Read the model definition and answer for the solid it produces. Units are mm, in the model's axes. A direction names the side the tool comes from. Give positions to 0.01 mm unless a question says otherwise; leave off trailing zeros. Order: outer loops, then holes, each group sorted by start corner. A loop starts at its lowest first (then second) coordinate and runs counter-clockwise, first axis right, second up. Notation, with made-up numbers: (44.25, -3.75) - (103.25, -3.75) arc R20 cw to (103.25, 25.25) - close; hole circle Ø4 at (71.25, -36). An arc over 180 degrees is marked (long way). Use a Markdown table: item, result. Add a question column.
1. Consider L1, parallel to Z at x = 25, y = 6.56; L2, parallel to Z at x = 13.5, y = 30.5; L3, parallel to Y at x = 27.5, z = -15 (3 decimals). Determine where each line is inside the solid, lowest interval first.
2. Which of the six approach directions +Z, -Z, +X, -X, +Y, -Y give full straight-line access (tool end or side, diameter ignored) to faces 1 (the flat face through (20, 8, -20)), 2 (the flat face through (18, 0, -27)), 3 (the flat face through (0, 53, -15))?
3. A cutting plane is placed at B-B on y = 15.06. Determine the outline of the cut face in (x, z) (3 decimals).
4. A cutting plane is placed at D-D on z = -3. Determine the outline of the cut face in (x, y).
5. For a pull along Z with two mould halves and no side action, classify faces 4 (the flat face through (25, -8, -8.025)), 5 (the flat face through (-19.27, 105.94, -14.79)), 6 (the cylindrical face through (25.07, 15.171, -12.477)) as released by +Z, released by -Z, zero draft, split by the parting line, or undercut.
6. A cutting plane is placed at C-C on x = 24. Determine the outline of the cut face in (y, z) (3 decimals), and give its area (3 significant figures).
7. Flat-ended cylindrical pins translate along their axes: P1, Ø10, axis at x = 14, y = 11.5, coming from the +Z side; P2, Ø10, axis at y = 104, z = -26.5, coming from the -X side; P3, Ø7.5, axis at y = 9, z = -17, coming from the -X side; P4, Ø7.5, axis at y = 23.56, z = -15, coming from the -X side. Find the tip coordinate at first contact, or state that the pin passes through.
8. A cutting plane is placed at A-A on z = -15. State how many separate pieces and enclosed holes the cut face has, and give its area (3 significant figures).
Autodesk Inventor part; units mm, degrees
ref_plane "YZ Plane" through (0, 0, 0) normal (1, 0, 0) x (0, 1, 0)
ref_plane "XZ Plane" through (0, 0, 0) normal (0, 1, 0) x (-1, 0, 0)
ref_plane "XY Plane" through (0, 0, 0) normal (0, 0, 1) x (1, 0, 0)
sketch "Sketch1" plane through (0, 0, 0) normal (0, 0, 1) x (1, 0, 0)
  line L0 (0, 0) -> (25, 0)
  line L1 (25, 0) -> (25, 40)
  line L2 (25, 40) -> (0, 40)
  line L3 (0, 40) -> (0, 0)
  dimension "d1" = 25
  dimension "d2" = 40
  dimension "d3" = 25
extrude "Extrusion1" add sketch "Sketch1" against normal blind 30
sketch "Sketch2" plane through (25, 0, 0) normal (1, 0, 0) x (0, 0, -1)
  line L0 (0, 0) -> (30, 0)
  circle A0 centre (15, 6.56) radius 2.46
extrude "Extrusion2" cut sketch "Sketch2" against normal blind 30
sketch "Sketch3" plane through (0, 0, 0) normal (-1, 0, 0) x (0, 0, 1)
  line L0 (0, 0) -> (-30, 0)
  line L1 (-25.05, 0) -> (-4.95, 0)
  line L2 (-4.95, 0) -> (-4.95, 33.12)
  line L3 (-4.95, 33.12) -> (-25.05, 33.12)
  line L4 (-25.05, 33.12) -> (-25.05, 0)
  dimension "d11" = 20.1
extrude "Extrusion3" cut sketch "Sketch3" against normal blind 20
sketch "Sketch4" plane through (0, 0, 0) normal (0, -1, 0) x (1, 0, 0)
  line L0 (20, -4.95) -> (20, -25.05)
  line L1 (20, -15) -> (25, -15)
  line L2 (25, 0) -> (25, -30)
  line L3 (20, -8.025) -> (25, -8.025)
  line L4 (25, -8.025) -> (25, -21.975)
  line L5 (25, -21.975) -> (20, -21.975)
  line L6 (20, -21.975) -> (20, -8.025)
  line L7 (20, -8.025) -> (25, -21.975) construction
  line L8 (25, -8.025) -> (20, -21.975) construction
  line L9 (25, -12.54) -> (25, -17.46)
  point P0 (0, 0)
  point P1 (22.5, -15)
  dimension "d14" = 13.95
extrude "Extrusion4" add sketch "Sketch4" along normal blind 15
sketch "Sketch5" plane through (20, 0, 0) normal (-1, 0, 0) x (0, 0, 1)
  circle A0 centre (-15, 6.56) radius 2.46
  circle A1 centre (-15, 6.56) radius 4.7025
  circle A2 centre (-15, 6.56) radius 2.46
  circle A3 centre (-15, 6.56) radius 2.46
  point P0 (0, 0)
  dimension "d17" = 9.405
extrude "Extrusion5" cut sketch "Sketch5" against normal blind 2.1
sketch "Sketch6" plane through (25, 0, 0) normal (1, 0, 0) x (0, 0, -1)
  circle A0 centre (15, 6.56) radius 4.7025
  line L0 (15, 6.56) -> (15, 23.56)
  circle A1 centre (15, 23.56) radius 2.46
  point P0 (0, 0)
  dimension "d20" = 17
  dimension "d21" = 4.92
extrude "Extrusion6" cut sketch "Sketch6" against normal blind 10 contours A1
sketch "Sketch7" plane through (20, 0, 0) normal (-1, 0, 0) x (0, 0, 1)
  circle A0 centre (-15, 23.56) radius 2.46
  circle A1 centre (-15, 23.56) radius 4.7025
  point P0 (0, 0)
  dimension "d24" = 9.405
extrude "Extrusion7" cut sketch "Sketch7" against normal blind 2.1
sketch "Sketch9" plane through (25, 0, 0) normal (1, 0, 0) x (0, 0, -1)
  circle A0 centre (15, 6.56) radius 2.46
  circle A1 centre (15, 6.56) radius 2.46
  circle A2 centre (15, 23.56) radius 2.46
  circle A3 centre (15, 23.56) radius 2.46
  line L0 (30, 40) -> (30, 0)
  line L1 (30, 0) -> (30, 40)
  line L2 (30, 40) -> (0, 40)
  line L3 (0, 40) -> (0, 0)
  line L4 (0, 0) -> (8.025, 0)
  line L5 (21.975, 0) -> (21.975, -15)
  line L6 (21.975, -15) -> (8.025, -15)
  line L7 (8.025, -15) -> (8.025, 0)
  line L8 (0, 0) -> (8.025, 0)
  line L9 (21.975, 0) -> (30, 0)
extrude "Extrusion8" add sketch "Sketch9" along normal blind 5
sketch "Sketch10" plane through (0, 40, 0) normal (0, 1, 0) x (1, 0, 0)
  line L0 (0, 30) -> (30, 30)
  line L1 (30, 0) -> (0, 0)
  line L2 (0, 30) -> (30, 30)
  line L3 (30, 30) -> (30, 0)
  line L4 (30, 0) -> (0, 0)
  line L5 (0, 0) -> (0, 30)
extrude "Extrusion9" add sketch "Sketch10" along normal blind 30
sketch "Sketch12" plane through (30, 0, 0) normal (1, 0, 0) x (0, 0, -1)
  circle A0 centre (15, 6.56) radius 2.46
  line L0 (15, 6.56) -> (15, 15.06)
  circle A1 centre (15, 15.06) radius 2.525
  point P0 (0, 0)
  dimension "d31" = 8.5
  dimension "d33" = 5.05
extrude "Extrusion10" cut sketch "Sketch12" against normal blind 30 contours A1
sketch "Sketch14" plane through (0, 0, 0) normal (0, 0, 1) x (1, 0, 0)
  line L0 (30, 70) -> (0, 70)
  line L1 (0, 70) -> (0, 85)
  line L2 (-15, 100) -> (-23, 100)
  line L3 (30, 0) -> (30, 70)
  line L4 (30, 100) -> (30, 70)
  arc A0 (0, 85) -> (-15, 100) centre (-15, 85) ccw
  line L5 (-23, 120) -> (15, 120)
  line L6 (-20.5, 118) -> (-18, 110)
  line L7 (-20.5, 118) -> (-23, 120)
  line L8 (-20.5, 102) -> (-18, 110)
  line L9 (-20.5, 102) -> (-23, 100)
  line L10 (30, 105) -> (15, 120)
  line L11 (30, 105) -> (30, 100)
  point P0 (0, 0)
  point P1 (0, 100)
  dimension "d47" = 30
  dimension "d54" = 15
  dimension "d60" = 20
extrude "Extrusion12" add sketch "Sketch14" against normal blind 30
sketch "Sketch15" plane through (0, 0, -25.05) normal (-1, 0, 0) x (0, 0, 1)
  line L0 (0, 33.12) -> (20.1, 33.12)
  line L1 (20.1, 33.12) -> (20.1, 0)
  line L2 (0, 33.12) -> (20.1, 33.12)
  line L3 (20.1, 33.12) -> (20.1, 31.1)
  line L4 (20.1, 31.1) -> (0, 31.1)
  line L5 (0, 31.1) -> (0, 33.12)
  point P0 (25.05, 0)
  dimension "d57" = 2.02
extrude "Extrusion13" add sketch "Sketch15" against normal blind 20
properties part number "16mm_x_30mm"
Output values:
| question | item | result |
|---|---|---|
| 1 | L1 | -30 to -17.46, -12.54 to 0 |
| 1 | L2 | -30 to -25.05, -4.95 to 0 |
| 1 | L3 | -15 to 4.1, 9.02 to 12.535, 17.585 to 21.1, 26.02 to 107.5 |
| 2 | face 1 | -X, -Y |
| 2 | face 2 | -Z, +X, -X, -Y |
| 2 | face 3 | +Z, -Z, -X, -Y |
| 3 | outline | (0, -30) - (30, -30) - (30, -17.525) - (20, -17.525) - (20, -25.05) - (0, -25.05) - close; (0, -4.95) - (20, -4.95) - (20, -12.475) - (30, -12.475) - (30, 0) - (0, 0) - close |
| 4 | outline | (-23, 100) - (-15, 100) arc R15 cw to (0, 85) - (0, 0) - (30, 0) - (30, 105) - (15, 120) - (-23, 120) - (-20.5, 118) - (-18, 110) - (-20.5, 102) - close |
| 5 | face 4 | released by +Z |
| 5 | face 5 | zero draft |
| 5 | face 6 | undercut |
| 6 | outline | (-15, -21.975) - (0, -21.975) - (0, -30) - (111, -30) - (111, 0) - (0, 0) - (0, -8.025) - (-15, -8.025) - close; hole circle Ø4.92 at (6.56, -15); hole circle Ø5.05 at (15.06, -15); hole circle Ø4.92 at (23.56, -15) |
| 6 | area | 3,480 mm² |
| 7 | P1 | z = 0 |
| 7 | P2 | x = -23 |
| 7 | P3 | x = 20 |
| 7 | P4 | x = 22.1 |
| 8 | separate pieces | 4 |
| 8 | enclosed holes | 0 |
| 8 | area | 3,290 mm² |
